from build123d import *

# Parameters (mm, degrees)
SKETCH1_W           = 20
SKETCH1_H           = 40
BOSS_EXTRUDE1_DEPTH = 8.7
SKETCH2_W           = 20
SKETCH2_H           = 40
BOSS_EXTRUDE2_DEPTH = 28.5
SKETCH3_R           = 2.25
BOSS_EXTRUDE3_DEPTH = 2.5
SKETCH4_R           = 2.794
BOSS_EXTRUDE4_DEPTH = 5
BOSS_EXTRUDE6_DEPTH = 6.9596
SKETCH10_R          = 6.30555
BOSS_EXTRUDE7_DEPTH = 0.889
CUT_EXTRUDE1_DEPTH  = 2.8956
SKETCH15_R          = 3.424566538
CUT_EXTRUDE4_DEPTH  = 20


with BuildPart() as part:
    # Sketch1 → Boss-Extrude1 (new body)
    with BuildSketch(Plane.XY):
        with Locations((10, 20)):
            Rectangle(SKETCH1_W, SKETCH1_H)
    extrude(amount=BOSS_EXTRUDE1_DEPTH)

    # Sketch2 → Boss-Extrude2 (add)
    with BuildSketch(Plane(origin=(0, 0, 0), x_dir=(-1, 0, 0), z_dir=(0, 0, -1))):
        with Locations((-10, 20)):
            Rectangle(SKETCH2_W, SKETCH2_H)
    extrude(amount=BOSS_EXTRUDE2_DEPTH)

    # Sketch3 → Boss-Extrude3 (add)
    with BuildSketch(Plane.XY):
        Polygon((19, 0), (19, -7.25), (1, -7.25), (1, 0), (0, 0), (0, 40), (1, 40), (1, 47.25), (19, 47.25), (19, 40), (20, 40), (20, 0), align=None)
        with Locations((5, -4.75)):
            Circle(SKETCH3_R, mode=Mode.SUBTRACT)
        with Locations((15, -4.75)):
            Circle(SKETCH3_R, mode=Mode.SUBTRACT)
        with Locations((5, 44.75)):
            Circle(SKETCH3_R, mode=Mode.SUBTRACT)
        with Locations((15, 44.75)):
            Circle(SKETCH3_R, mode=Mode.SUBTRACT)
    extrude(amount=BOSS_EXTRUDE3_DEPTH)

    # Sketch4 → Boss-Extrude4 (add)
    with BuildSketch(Plane.XY.offset(8.7)):
        with Locations((10, 29.6)):
            Circle(SKETCH4_R)
    extrude(amount=BOSS_EXTRUDE4_DEPTH)

    # Sketch9 → Boss-Extrude6 (add)
    with BuildSketch(Plane(origin=(0, 0, -28.5), x_dir=(-1, 0, 0), z_dir=(0, 0, -1))):
        Polygon((-13.1115, 40), (-6.8885, 40), (-7.714, 45.842), (-12.286, 45.842), align=None)
    extrude(amount=-BOSS_EXTRUDE6_DEPTH)

    # Sketch10 → Boss-Extrude7 (add)
    with BuildSketch(Plane.XY.offset(8.7)):
        with Locations((10, 29.6)):
            Circle(SKETCH10_R)
    extrude(amount=BOSS_EXTRUDE7_DEPTH)

    # Sketch11 → Cut-Extrude1 (cut)
    with BuildSketch(Plane(origin=(0, 0, -28.5), x_dir=(-1, 0, 0), z_dir=(0, 0, -1))):
        Polygon((-12.286, 45.842), (-7.714, 45.842), (-6.8885, 40), (-13.1115, 40), align=None)
    extrude(amount=-CUT_EXTRUDE1_DEPTH, mode=Mode.SUBTRACT)

    # Sketch15 → Cut-Extrude4 (cut)
    with BuildSketch(Plane(origin=(20, 0, 0), x_dir=(0, 0, -1), z_dir=(1, 0, 0))):
        with Locations((11.945832328, 29.752689179)):
            Circle(SKETCH15_R)
    extrude(amount=-CUT_EXTRUDE4_DEPTH, mode=Mode.SUBTRACT)


solid = part.part
Part model, mm, in its own coordinate system. A direction names the side the tool comes from. Coordinates: 2 decimals unless noted, no trailing zeros. Order: outer loops, then holes, each group sorted by start corner. A loop starts at its lowest first (then second) coordinate and runs counter-clockwise, first axis right, second up. Notation, with made-up numbers: (4, 3.25) - (15, 3.25) arc R8 ccw to (15, 11.25) - close; hole circle Ø1 at (21.25, 36.25). An arc over 180 degrees is marked (long way). Use CSV: the item, a comma, the result in double quotes.
Item 1: Saw through at C-C on y = 44.75. Give the cut face in (x, z), and give its area (3 significant figures).
Solved:
outline,"(1, 0) - (2.75, 0) - (2.75, 2.5) - (1, 2.5) - close; (7.25, 0) - (12.75, 0) - (12.75, 2.5) - (7.25, 2.5) - close; (7.56, -25.6) - (12.44, -25.6) - (12.44, -21.54) - (7.56, -21.54) - close; (17.25, 0) - (19, 0) - (19, 2.5) - (17.25, 2.5) - close"
area,"42.3 mm²"
Item 2: Probe probe 1 along Y at (x, z) = (15, 0.55); probe 2 along Z at (x, y) = (14.5, 1.5); probe 3 along Y at (x, z) = (4.75, -7). List the from-to ranges inside material, lowest first.
Solved:
probe 1,"y = -7.25 to -7, -2.5 to 42.5, 47 to 47.25"
probe 2,"z = -28.5 to 8.7"
probe 3,"y = 0 to 40"
Item 3: Saw through at B-B on y = -4.75. Give the cut face in (x, z).
Solved:
outline,"(1, 0) - (2.75, 0) - (2.75, 2.5) - (1, 2.5) - close; (7.25, 0) - (12.75, 0) - (12.75, 2.5) - (7.25, 2.5) - close; (17.25, 0) - (19, 0) - (19, 2.5) - (17.25, 2.5) - close"
Item 4: 3-axis set-ups, long thin cutter, end or side, ignore diameter. For faces 4 (the face through (19, 44, 1)), 5 (the face through (13, 28, 9.589)), 6 (the face through (10, 45.842, -24)): which of +Z, -Z, +X, -X, +Y, -Y reach the whole face in a straight line?
Solved:
face 4,"+Z, -Z, +X, +Y"
face 5,"+Z"
face 6,"-Z, +X, -X, +Y"
Item 5: Drop flat-ended pins along their axis: P1, Ø2, axis at y = 43, z = 1.5, coming from the +X side; P2, Ø6, axis at x = 15, y = 44.75, coming from the -Z side; P3, Ø2, axis at x = 6, y = -5, coming from the -Z side; P4, Ø8, axis at x = 4, z = 7.5, coming from the +Y side. Give the stop position or say it passes through.
Solved:
P1,"stops at x = 19"
P2,"stops at z = -25.6"
P3,"passes through"
P4,"stops at y = 40"
Item 6: Saw through at A-A on x = 14.5. Give the cut face in (y, z).
Solved:
outline,"(-7.25, 0) - (-6.94, 0) - (-6.94, 2.5) - (-7.25, 2.5) - close; (-2.56, 0) - (0, 0) - (0, -28.5) - (40, -28.5) - (40, 0) - (42.56, 0) - (42.56, 2.5) - (40, 2.5) - (40, 8.7) - (34.02, 8.7) - (34.02, 9.59) - (25.18, 9.59) - (25.18, 8.7) - (0, 8.7) - (0, 2.5) - (-2.56, 2.5) - close; (46.94, 0) - (47.25, 0) - (47.25, 2.5) - (46.94, 2.5) - close; hole circle Ø6.85 at (29.75, -11.95)"
Item 7: Mould opens along Y. For faces 1 (the face through (9.18, 35.85, 9.14)), 2 (the face through (17.146, -4.074, 1.232)), 3 (the face through (1, -4, 1)) say: +Y half, -Y half, draft (parallel to the pull), parting line (faces both ways), or undercut.
Solved:
face 1,"parting line"
face 2,"undercut"
face 3,"draft"
Item 8: Saw through at D-D on z = -11.5. Give the cut face in (x, y), and give its area (3 significant figures).
Solved:
outline,"(0, 0) - (20, 0) - (20, 26.36) - (0, 26.36) - close; (0, 33.15) - (20, 33.15) - (20, 40) - (0, 40) - close"
area,"664 mm²"
